Design review of the part shown in the three views and the two pictorial views. Dimensions are in mm from the part's minimum x, y and z. Round coordinates to 2 decimals unless told otherwise and drop trailing zeros. Loops run counter-clockwise (first coordinate to the right, second up) from the corner with the lowest first, then second, coordinate; pieces in that order, holes last. Notation, with made-up numbers: M 44.5,20 L 48.5,20 A10 ccw 48.5,24 Z; hole C -17.5,62.25 d8. An arc over 180 degrees is marked long. Return JSON: item names as keys, results as strings. Group by question number.
Q1. Consider section B-B (x = 53). State the section outline as (y, z) points.
Q2. To check wall thickness, follow line 1 along Z through (x, y) = (92.3, 0.7); line 2 along X through (y, z) = (0.15, 15); line 3 along Z through (x, y) = (22, 0.4). State the ranges of each line that lie inside material, in increasing order.
Q3. Consider section A-A (z = 35.5). State the section outline as (x, y) points, and give its area (3 significant figures).
Q4. Consider section C-C (z = 63.65). State the section outline as (x, y) points.
Q5. Consider section D-D (y = 1). State the section outline as (x, z) points, and give its area (3 significant figures).
Q6. Clearance check with a flat-ended pin moving along its axis: pin 1 Ø0.8 at (y, z) = (1, 20) entering from -X. State where the tip first meets the part, or that it passes through.
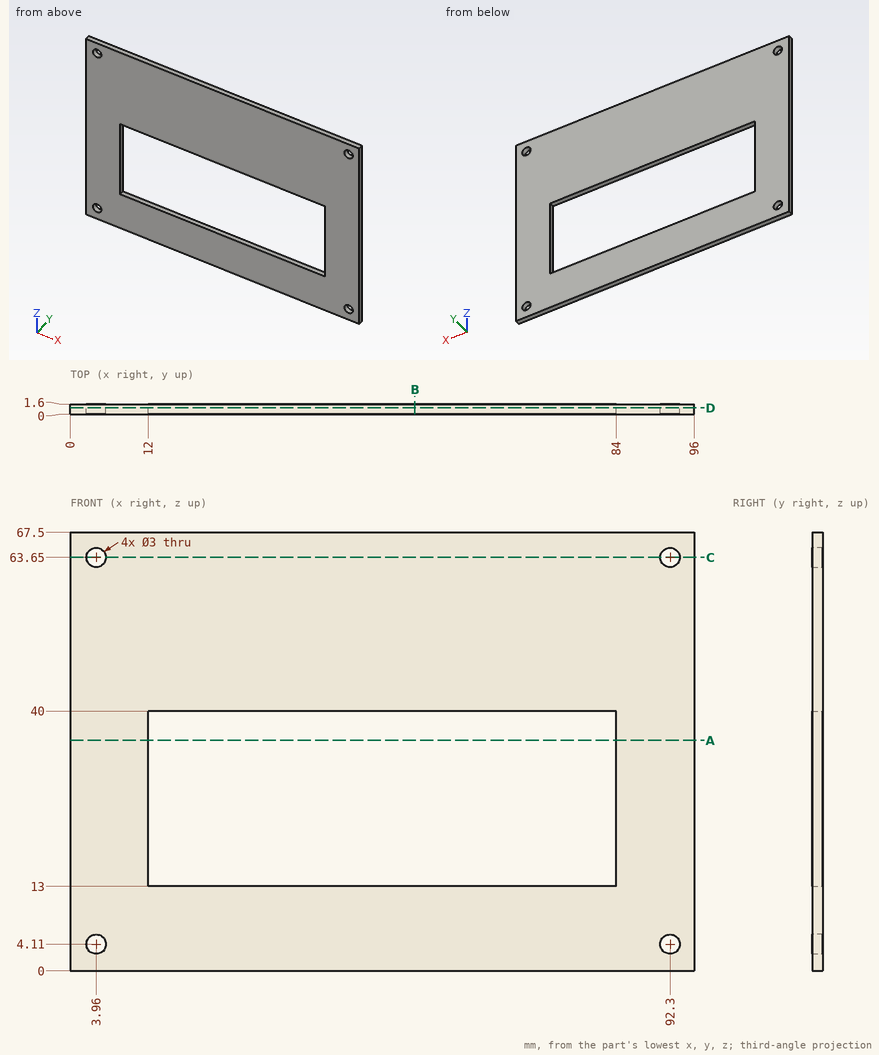
Values:
{
 "1": {"outline": "M 0,0 L 1.6,0 L 1.6,13 L 0,13 Z; M 0,40 L 1.6,40 L 1.6,67.5 L 0,67.5 Z"},
 "2": {"line 1": "z = 0 to 2.61, 5.61 to 62.15, 65.15 to 67.5", "line 2": "x = 0 to 12, 84 to 96", "line 3": "z = 0 to 13, 40 to 67.5"},
 "3": {"outline": "M 0,0 L 12,0 L 12,1.6 L 0,1.6 Z; M 84,0 L 96,0 L 96,1.6 L 84,1.6 Z", "area": "38.4 mm2"},
 "4": {"outline": "M 0,0 L 2.46,0 L 2.46,1.6 L 0,1.6 Z; M 5.46,0 L 90.8,0 L 90.8,1.6 L 5.46,1.6 Z; M 93.8,0 L 96,0 L 96,1.6 L 93.8,1.6 Z"},
 "5": {"outline": "M 0,0 L 96,0 L 96,67.5 L 0,67.5 Z; hole C 3.96,4.11 d3; hole C 3.96,63.65 d3; hole M 12,13 L 84,13 L 84,40 L 12,40 Z; hole C 92.3,4.11 d3; hole C 92.3,63.65 d3", "area": "4,510 mm2"},
 "6": {"pin 1": "stops at x = 0"}
}
